Build history of the part. All positions in model axes, mm. A direction names the side the tool comes from. Round coordinates to 2 decimals unless told otherwise and drop trailing zeros. Write each loop counter-clockwise with the first axis right and the second up, starting at its lowest first coordinate (ties: lowest second). Pieces come first, ordered by that corner, then holes. Notation, with made-up numbers: M 28,-23 L 40,-23 A20 cw 40,0 Z; hole C 65,-31 d7. An arc over 180 degrees is marked long. Write item = value, one per line.
from build123d import *

# Parameters (mm, degrees)
F1_DEPTH  = 6
F2_W      = 20
F2_H      = 5.42
F3_DEPTH  = 2
F4_R      = 2.25
F5_DEPTH  = 8.001
F6_R      = 3.75
F7_DEPTH  = 2
F8_W      = 60
F8_H      = 6
F9_DEPTH  = 6
F10_W     = 60
F10_H     = 6
F11_DEPTH = 20
F13_DEPTH = 60
F15_DEPTH = 20
F16_W     = 42
F16_H     = 5.42
F17_DEPTH = 2
F19_DEPTH = 20
F20_W     = 42
F20_H     = 5.42
F21_DEPTH = 2
F22_R     = 2.25
F23_DEPTH = 46.001
F24_R     = 2.25
F25_DEPTH = 8
F26_R     = 3.75
F27_DEPTH = 2
F28_R     = 3.75
F29_DEPTH = 2
F30_R     = 3.75
F31_DEPTH = 2
F32_SIZE  = 3


with BuildPart() as f1:
    # F0 (on Top) → F1 (new body)
    with BuildSketch(Plane.XY):
        Polygon((-30, 0), (-10, 0), (-10, -40), (0, -40), (10, -40), (10, 0), (30, 0), (30, 20), (0, 20), (-30, 20), align=None)
    extrude(amount=F1_DEPTH)

    # F2 (on face) → F3 (join)
    with BuildSketch(Plane.XY.offset(6)):
        Polygon((2.71, 0), (0, 0), (-2.71, 0), (-2.71, -40), (2.71, -40), align=None)
        Polygon((10, 12.71), (10, 10), (10, 7.29), (30, 7.29), (30, 12.71), align=None)
        with Locations((-20, 10)):
            Rectangle(F2_W, F2_H)
    extrude(amount=F3_DEPTH)

    # F4 (on face) → F5 (cut, through all)
    with BuildSketch(Plane(origin=(0, 0, 0), x_dir=(1, 0, 0), z_dir=(0, 0, -1))):
        with Locations((-20, -10)):
            Circle(F4_R)
        with Locations((0, 10)):
            Circle(F4_R)
        with Locations((0, 30)):
            Circle(F4_R)
        with Locations((20.741304, -10)):
            Circle(F4_R)
        with Locations((0, -10)):
            Circle(F4_R)
    extrude(amount=-F5_DEPTH, mode=Mode.SUBTRACT)

    # F6 (on face) → F7 (cut)
    with BuildSketch(Plane(origin=(0, 0, 0), x_dir=(1, 0, 0), z_dir=(0, 0, -1))):
        with Locations((0, 30)):
            Circle(F6_R)
        with Locations((0, 10)):
            Circle(F6_R)
        with Locations((20.741304, -10)):
            Circle(F6_R)
        with Locations((-20, -10)):
            Circle(F6_R)
        with Locations((0, -10)):
            Circle(F6_R)
    extrude(amount=-F7_DEPTH, mode=Mode.SUBTRACT)

    # F8 (on face) → F9 (join)
    with BuildSketch(Plane(origin=(0, 0, 0), x_dir=(1, 0, 0), z_dir=(0, 0, -1))):
        Polygon((-10, 0), (-10, 40), (-30, 0), align=None)
        Polygon((30, 0), (10, 40), (10, 0), align=None)
        with Locations((0, -23)):
            Rectangle(F8_W, F8_H)
    extrude(amount=-F9_DEPTH)

    # F10 (on face) → F11 (join)
    with BuildSketch(Plane.XY.offset(6)):
        Polygon((30, 0), (10, 0), (10, -40), (16, -28), (16, -6), (27, -6), align=None)
        Polygon((-10, -40), (-10, 0), (-30, 0), (-27, -6), (-16, -6), (-16, -28), align=None)
        with Locations((0, 23)):
            Rectangle(F10_W, F10_H)
    extrude(amount=F11_DEPTH)

    # F12 (on face) → F13 (join)
    with BuildSketch(Plane.YZ.offset(30)):
        Polygon((20, 13.29), (20, 16), (20, 18.71), (18, 18.71), (18, 13.29), align=None)
    extrude(amount=-F13_DEPTH)

    # F14 (on face) → F15 (join)
    with BuildSketch(Plane.YZ.offset(-10)):
        Polygon((0, 18.71), (0, 16), (0, 13.29), (2, 13.29), (2, 18.71), align=None)
    extrude(amount=-F15_DEPTH)

    # F16 (on face) → F17 (join)
    with BuildSketch(Plane.YZ.offset(-10)):
        with Locations((-19, 16)):
            Rectangle(F16_W, F16_H)
    extrude(amount=F17_DEPTH)

    # F18 (on face) → F19 (join)
    with BuildSketch(Plane(origin=(10, 0, 0), x_dir=(0, -1, 0), z_dir=(-1, 0, 0))):
        Polygon((0, 13.29), (0, 16), (0, 18.71), (-2, 18.71), (-2, 13.29), align=None)
    extrude(amount=-F19_DEPTH)

    # F20 (on face) → F21 (join)
    with BuildSketch(Plane(origin=(10, 0, 0), x_dir=(0, -1, 0), z_dir=(-1, 0, 0))):
        with Locations((19, 16)):
            Rectangle(F20_W, F20_H)
    extrude(amount=F21_DEPTH)

    # F22 (on face) → F23 (cut, through all)
    with BuildSketch(Plane(origin=(-16, 0, 0), x_dir=(0, -1, 0), z_dir=(-1, 0, 0))):
        with Locations((20, 16)):
            Circle(F22_R)
    extrude(amount=-F23_DEPTH, mode=Mode.SUBTRACT)

    # F24 (on face) → F25 (cut, through all)
    with BuildSketch(Plane(origin=(0, 26, 0), x_dir=(-1, 0, 0), z_dir=(0, 1, 0))):
        with Locations((-20, 16)):
            Circle(F24_R)
        with Locations((0, 16)):
            Circle(F24_R)
        with Locations((20, 16)):
            Circle(F24_R)
    extrude(amount=-F25_DEPTH, mode=Mode.SUBTRACT)

    # F26 (on face) → F27 (cut)
    with BuildSketch(Plane.YZ.offset(16)):
        with Locations((-20, 16)):
            Circle(F26_R)
    extrude(amount=-F27_DEPTH, mode=Mode.SUBTRACT)

    # F28 (on face) → F29 (cut)
    with BuildSketch(Plane(origin=(-16, 0, 0), x_dir=(0, -1, 0), z_dir=(-1, 0, 0))):
        with Locations((20, 16)):
            Circle(F28_R)
    extrude(amount=-F29_DEPTH, mode=Mode.SUBTRACT)

    # F30 (on face) → F31 (cut)
    with BuildSketch(Plane(origin=(0, 26, 0), x_dir=(-1, 0, 0), z_dir=(0, 1, 0))):
        with Locations((-20, 16)):
            Circle(F30_R)
        with Locations((0, 16)):
            Circle(F30_R)
        with Locations((20, 16)):
            Circle(F30_R)
    extrude(amount=-F31_DEPTH, mode=Mode.SUBTRACT)

    # F32
    f32_edges = [f1.edges().sort_by_distance(p)[0] for p in [
        (0, 26, 0),
        (30, 26, 13),
        (-30, 26, 13),
        (-30, 13, 0),
        (30, 13, 0),
        (20, -20, 0),
        (-20, -20, 0),
        (0, -40, 0),
        (0, 26, 26),
        (-21.5, -6, 26),
        (-16, -17, 26),
        (16, -17, 26),
        (21.5, -6, 26),
        (-13, -34, 26),
        (13, -34, 26),
    ]]
    chamfer(f32_edges, length=F32_SIZE)


solid = f1.part
1. Band-saw the part on C-C (y = 10). Count the separate pieces of the cut face and the enclosed holes in it, plus the area to 3 significant figures.
Responses:
separate_pieces = 4
enclosed_holes = 0
area = 314 mm²
2. Band-saw the part on A-A (y = 19). List the corners of the cut face in (x, z), plus the area to 3 significant figures.
Responses:
outline = M -30,3 L -27,0 L 27,0 L 30,3 L 30,6 L -30,6 Z; M -30,13.29 L 30,13.29 L 30,18.71 L -30,18.71 Z; hole C -20,16 d4.5; hole C 0,16 d4.5; hole C 20,16 d4.5
area = 628 mm²
3. Tool access for faces 1 (the face through (15.014, -18.27, 12.673)), 2 (the face through (9, -13, 13.29)), 3 (the face through (-19, 2, 16)), 4 (the face through (-14, -22, 14)), 5 (the face through (-21, -5, 24)): list every direction of +Z, -Z, +X, -X, +Y, -Y with a clear straight run to the whole face (end or side of a thin tool).
Responses:
face_1 = +X
face_2 = none
face_3 = +Z, +X, -X
face_4 = -X
face_5 = +Z, -X, -Y
4. Mould opens along Y. For faces 6 (the face through (0, 3, 6)), 7 (the face through (28, 25, 14)), 8 (the face through (-19.19, 25.01, 12.34)) say: pulls with the +Y half, pulls with the -Y half, needs draft (parallel to the pull), parting line crosses it, or undercut.
Responses:
face_6 = undercut
face_7 = pulls with the +Y half
face_8 = needs draft
5. Band-saw the part on B-B (z = 11). List the corners of the cut face in (x, y).
Responses:
outline = M -30,0 L -27,-6 L -16,-6 L -16,-28 L -10,-40 L -10,0 Z; M -30,20 L 30,20 L 30,23 L 27,26 L -27,26 L -30,23 Z; M 10,-40 L 16,-28 L 16,-6 L 27,-6 L 30,0 L 10,0 Z
6. Flat gauge pins, fed straight in: pin 1 (4.5 mm diameter, centred on y = -19, z = 15.5, fed in from -X); pin 2 (6 mm diameter, centred on x = 10, y = 18, fed in from +Z); pin 3 (4 mm diameter, centred on x = -20, z = 16, fed in from +Y); pin 4 (10 mm diameter, centred on x = 1, z = 20.5, fed in from -Y). Where does each tip first touch, or does it go through?
Responses:
pin_1 = -14
pin_2 = 26
pin_3 = 2
pin_4 = 18
7. Probe probe 1 along Z at (x, y) = (15, 19); probe 2 along X at (y, z) = (-7, 9); probe 3 along Y at (x, z) = (18, 14.5). List the from-to ranges inside material, lowest first.
Responses:
probe_1 = 0 to 6, 13.29 to 18.71
probe_2 = -16 to -10, 10 to 16
probe_3 = -6 to 2, 18 to 24
